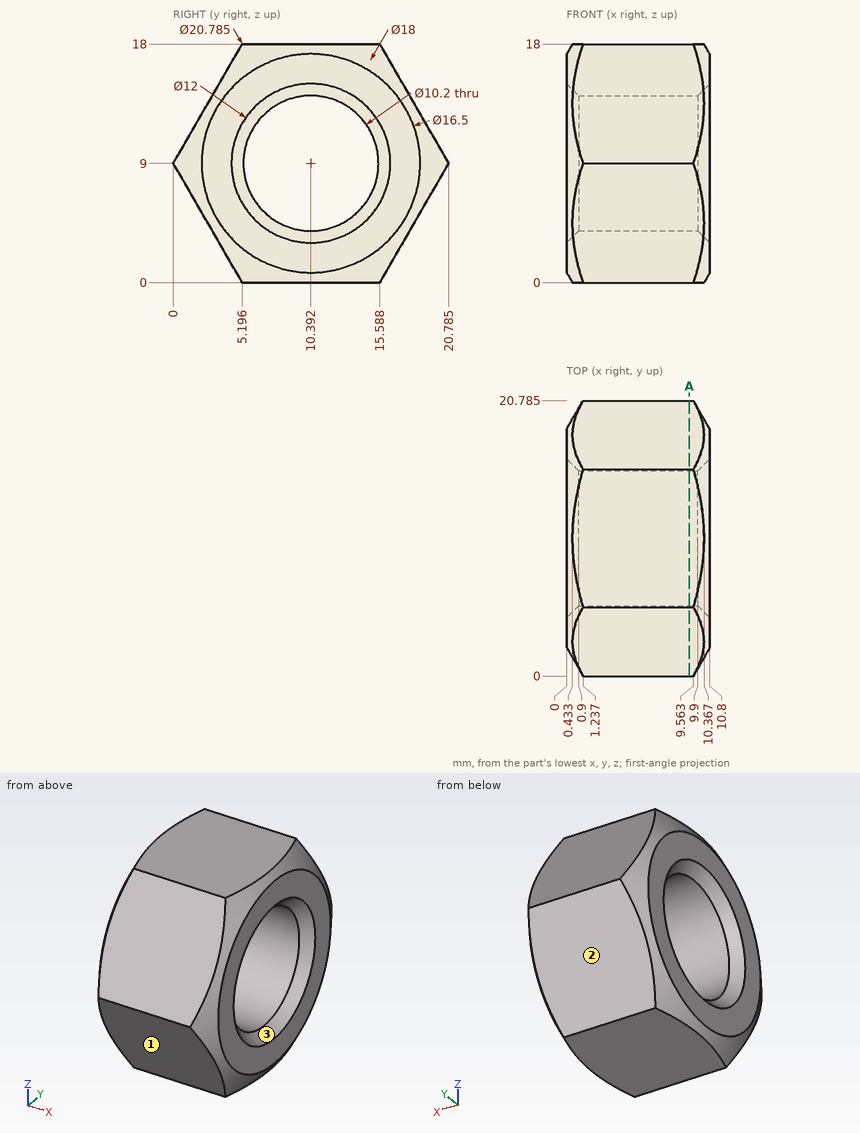
Job drawing, mm, ordinate dimensions from the low corner. One solid piece. Round coordinates to 2 decimals unless told otherwise and drop trailing zeros. Write each loop counter-clockwise with the first axis right and the second up, starting at its lowest first coordinate (ties: lowest second). Pieces come first, ordered by that corner, then holes. Notation, with made-up numbers: M 2,2.5 L 50,2.5 A28 cw 50,22.5 Z; hole C -20,8 d1. An arc over 180 degrees is marked long. Return JSON: item names as keys, results as strings. Group by question number.
(1) Saw through at A-A on x = 9.25. Write the cut outline in (y, z) (1 decimal), then the cut area to 3 significant figures.
(2) Drill centre lines: probe 1 along Z at (x, y) = (9.5, 11.5); probe 2 along Y at (x, z) = (10, 8) (1 decimal); probe 3 along Z at (x, y) = (8, 12.5) (1 decimal). Where is each one in solid material? Low to high.
(3) Two-plate mould, pull along Y, no slides. Class the marked faces 1, 2 and 3: +Y half, -Y half, draft (parallel to the pull), parting line (faces both ways), or undercut.
(4) Pin check, flat tip, straight feed: pin 1 Ø4 at (x, z) = (7, 10) entering from -Y. Stop position of the tip, or through.
Returned:
{
 "1": {"outline": "M 0,9 L 5.2,0 L 15.6,0 L 20.8,9 L 15.6,18 L 5.2,18 Z; hole C 10.4,9 d10.2", "area": "199 mm²"},
 "2": {"probe 1": "0 to 4.02, 13.98 to 18", "probe 2": "0.8 to 5.3, 15.5 to 20", "probe 3": "0 to 4.4, 13.6 to 18"},
 "3": {"face 1": "-Y half", "face 2": "+Y half", "face 3": "undercut"},
 "4": {"pin 1": "y = 0"}
}
